The figure shows three views and two pictorial views of one solid part (mm, origin at its lowest corner). Answer the questions. A direction names the side the tool comes from. Give positions to 0.01 mm unless a question says otherwise; leave off trailing zeros. Order: outer loops, then holes, each group sorted by start corner. A loop starts at its lowest first (then second) coordinate and runs counter-clockwise, first axis right, second up. Notation, with made-up numbers: (86, 13) - (91, 13) arc R19 ccw to (91, 42) - close; hole circle Ø1 at (6.5, 1). An arc over 180 degrees is marked (long way). Answer as a JSON object with one key per item and string values. Group by question number.
Q1. Consider line 1 (X direction, y = 20, z = 6.5); line 2 (Y direction, x = 3.3, z = 9.3); line 3 (Y direction, x = 13.3, z = 8.2). Determine where each line is inside the solid, lowest interval first.
Q2. For the marked faces 5, 6 and 7, determine the directions among +Z, -Z, +X, -X, +Y, -Y from which every point of the face is accessible in a straight line to the end or side of a thin tool.
Q3. A cutting plane is placed at B-B, the plane y = 20. Give the vertices of the cut face in (x, z).
Q4. A cutting plane is placed at C-C, the plane z = 8.5. Give the vertices of the cut face in (x, y), and give its area (3 significant figures).
Q5. A cutting plane is placed at D-D, the plane z = 6.5. Give the vertices of the cut face in (x, y).
Q6. Given pin 1 (1.4 mm diameter, centred on y = 18, z = 1, fed in from +X); pin 2 (2 mm diameter, centred on x = 5, y = 17.5, fed in from -Z); pin 3 (3 mm diameter, centred on y = 4.5, z = 4.5, fed in from -X); pin 4 (0.6 mm diameter, centred on x = 3, z = 9, fed in from +Y), each flat-ended and moving along its own axis, determine where each tip first touches the part or whether it passes through.
Q7. The mould has two halves that part along Y. Classify the marked faces 1, 2, 3 and 4: released by +Y, released by -Y, zero draft, split by the parting line, or undercut.
Q8. A cutting plane is placed at A-A, the plane x = 14.8. Give the vertices of the cut face in (y, z).
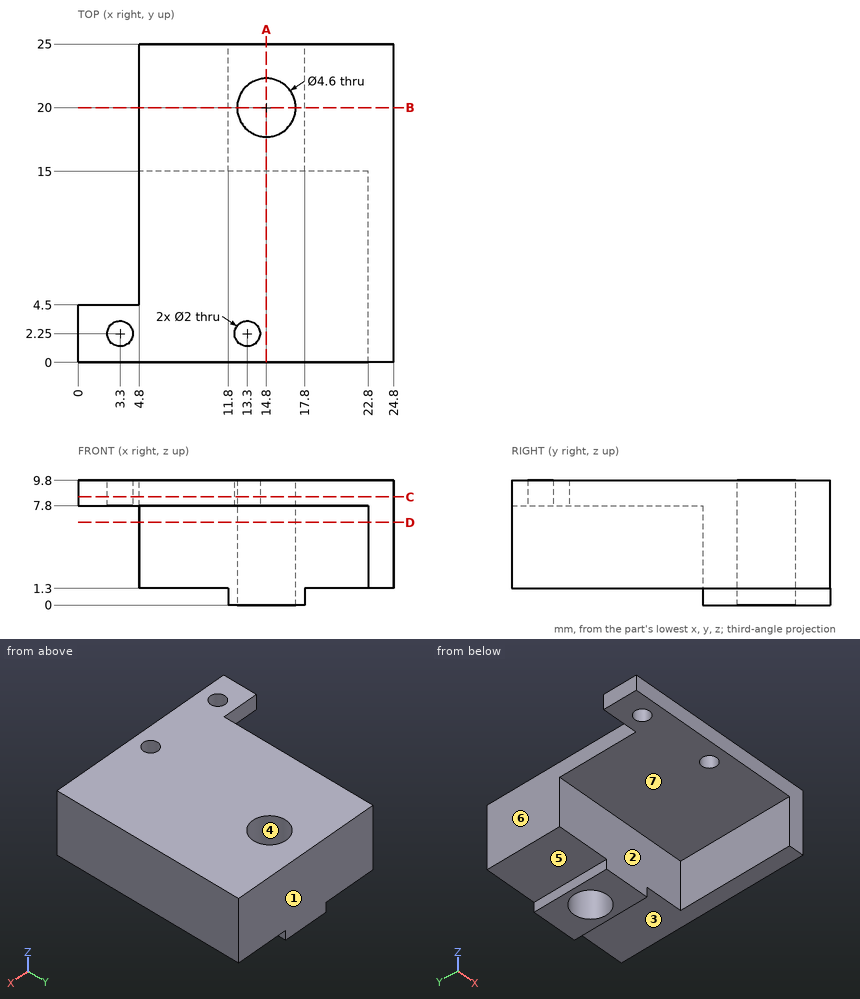
Reply:
{
 "1": {"line 1": "x = 4.8 to 12.5, 17.1 to 24.8", "line 2": "y = 0 to 1.25, 3.25 to 4.5", "line 3": "y = 0 to 1.25, 3.25 to 18.26, 21.74 to 25"},
 "2": {"face 5": "-Z, -X, +Y, -Y", "face 6": "+Z, -Z, -X, +Y", "face 7": "-Z, -X, -Y"},
 "3": {"outline": "(4.8, 1.3) - (11.8, 1.3) - (11.8, 0) - (12.5, 0) - (12.5, 9.8) - (4.8, 9.8) - close; (17.1, 0) - (17.8, 0) - (17.8, 1.3) - (24.8, 1.3) - (24.8, 9.8) - (17.1, 9.8) - close"},
 "4": {"outline": "(0, 0) - (24.8, 0) - (24.8, 25) - (4.8, 25) - (4.8, 4.5) - (0, 4.5) - close; hole circle Ø2 at (3.3, 2.25); hole circle Ø2 at (13.3, 2.25); hole circle Ø4.6 at (14.8, 20)", "area": "499 mm^2"},
 "5": {"outline": "(4.8, 15) - (22.8, 15) - (22.8, 0) - (24.8, 0) - (24.8, 25) - (4.8, 25) - close; hole circle Ø4.6 at (14.8, 20)"},
 "6": {"pin 1": "stops at x = 24.8", "pin 2": "stops at z = 1.3", "pin 3": "stops at x = 22.8", "pin 4": "stops at y = 4.5"},
 "7": {"face 1": "released by +Y", "face 2": "released by -Y", "face 3": "zero draft", "face 4": "undercut"},
 "8": {"outline": "(0, 7.8) - (15, 7.8) - (15, 0) - (17.7, 0) - (17.7, 9.8) - (0, 9.8) - close; (22.3, 0) - (25, 0) - (25, 9.8) - (22.3, 9.8) - close"}
}
